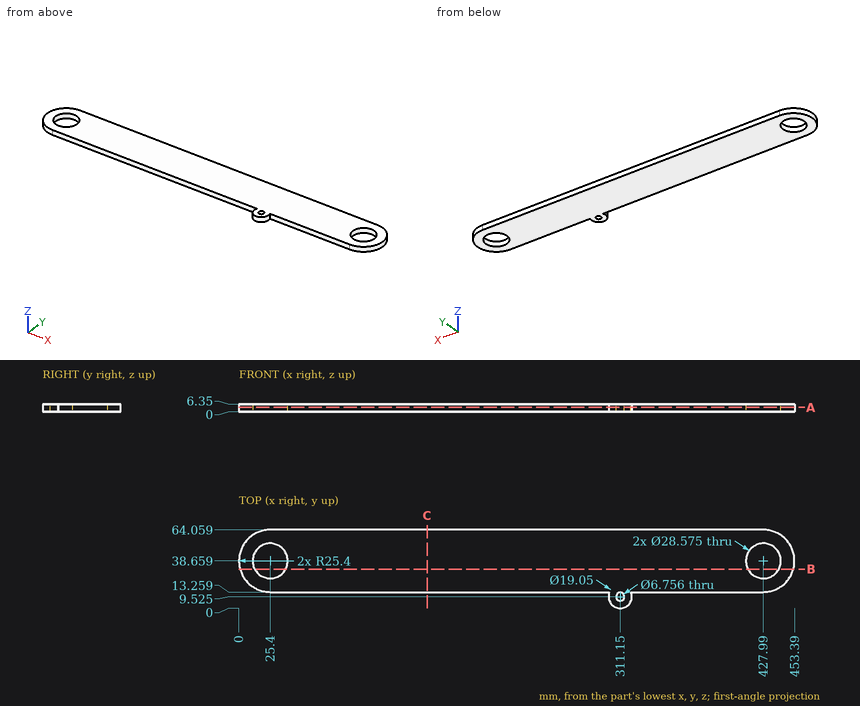
Answer from the drawing. Dimensions are ordinates in mm from the lowest x, y and z of the part. Give positions to 0.01 mm unless a question says otherwise; leave off trailing zeros. Write each loop counter-clockwise with the first axis right and the second up, starting at its lowest first coordinate (ties: lowest second). Pieces come first, ordered by that corner, then holes. Notation, with made-up numbers: (42, -30) -> (55, -30) arc R31 ccw to (55, 0) -> close; hole circle Ø4 at (5, -24.75). An arc over 180 degrees is marked (long way). One line per question, with ' | ' between items. Start each with the question number.
1. Section C-C (x = 153.5) is taken. Determine the outline of the cut face in (y, z).
2. Section B-B (y = 32) is taken. Determine the outline of the cut face in (x, z), plus the area to 3 significant figures.
3. Given pin 1 Ø2 at (x, z) = (138.5, 2.5) entering from -Y; pin 2 Ø1 at (y, z) = (48.5, 2) entering from +X, each flat-ended and moving along its own axis, determine where each tip first touches the part or whether it passes through.
4. Section A-A (z = 3.5) is taken. State how many separate pieces and enclosed holes the cut face has, plus the area to 3 significant figures.
5. Find the intervals of material crossed by probe 1 along Y at (x, z) = (25.4, 2); probe 2 along X at (y, z) = (39.5, 2.75); probe 3 along X at (y, z) = (42, 2.75), in increasing order.
Response values:
1) outline: (13.26, 0) -> (64.06, 0) -> (64.06, 6.35) -> (13.26, 6.35) -> close
2) outline: (0.89, 0) -> (12.76, 0) -> (12.76, 6.35) -> (0.89, 6.35) -> close; (38.04, 0) -> (415.35, 0) -> (415.35, 6.35) -> (38.04, 6.35) -> close; (440.63, 0) -> (452.5, 0) -> (452.5, 6.35) -> (440.63, 6.35) -> close | area: 2,550 mm2
3) pin 1: y = 13.26 | pin 2: x = 451.61
4) separate pieces: 1 | enclosed holes: 3 | area: 21,400 mm2
5) probe 1: 13.26 to 24.37, 52.95 to 64.06 | probe 2: 0.01 to 11.14, 39.66 to 413.73, 442.25 to 453.38 | probe 3: 0.22 to 11.51, 39.29 to 414.1, 441.88 to 453.17
